Geometry check sheet. Reference: the model listing, model coordinates, mm. Face numbers are marked on the shaded views. A direction names the side the tool comes from. Round coordinates to 2 decimals unless told otherwise and drop trailing zeros. Order: outer loops, then holes, each group sorted by start corner. A loop starts at its lowest first (then second) coordinate and runs counter-clockwise, first axis right, second up. Notation, with made-up numbers: (20.5, -31.5) - (37.5, -31.5) arc R15 ccw to (37.5, -9.5) - close; hole circle Ø10 at (2.5, 82). An arc over 180 degrees is marked (long way). Use a Markdown table: item, result. Add a question column.
(1) Section check A-A on x = 28.25. Record the boundary of the cut face in (y, z) (3 decimals), then the cut area to 3 significant figures.
(2) Section check C-C on z = 13. Record the boundary of the cut face in (x, y), then the cut area to 3 significant figures.
(3) Section check D-D on z = 2.5. Record the boundary of the cut face in (x, y).
(4) Gauge pin test, flat ends, axial feed: P1, Ø3.5, axis at y = 15.5, z = -2, coming from the -X side; P2, Ø10.5, axis at y = -5.5, z = 20, coming from the -X side; P3, Ø6, axis at y = -18, z = 2, coming from the +X side; P4, Ø3, axis at x = 0, y = 0, coming from the -Z side. Record the tip position at first contact, or that the pin passes through.
(5) Access from +Z, -Z, +X, -X, +Y, -Y to the whole of each face (thin tool, end or side, straight path). Record for the marked faces 1, 2, 3 and 4.
(6) Thickness scan on line 1 along Y through (x, z) = (0, -1.3) (3 decimals); line 2 along Z through (x, y) = (-16.5, -10); line 3 along X through (y, z) = (-1, 4). Record the ranges inside material, lowest first. Write a range as [from, to].
```python
from build123d import *

# Parameters (mm, degrees)
F0_R     = 1
F0_R_2   = 1.25
F0_R_3   = 4.2
F0_R_4   = 1.275
F0_W     = 11.2
F0_H     = 6.2
F1_DEPTH = 3
F4_W     = 10.83598
F4_H     = 10.83598
F5_DEPTH = 40


with BuildPart() as f1:
    # F0 (on Top) → F1 (new body)
    with BuildSketch(Plane.XY):
        with BuildLine():
            ThreePointArc((26.336773, -20), (31.34153, -10.551499), (33.070011, 0))
            ThreePointArc((33.070011, 0), (14.700772, 29.622845), (-20, 26.336773))
            Line((-20, 26.336773), (-20, -20))
            Line((-20, -20), (26.336773, -20))
        make_face()
        with Locations((-15, 3e-06)):
            Circle(F0_R, mode=Mode.SUBTRACT)
        Circle(F0_R_2, mode=Mode.SUBTRACT)
        with Locations((0, 19)):
            Circle(F0_R_3, mode=Mode.SUBTRACT)
        with Locations((0, 28.25)):
            Circle(F0_R_4, mode=Mode.SUBTRACT)
        with Locations((11.580758, 16.082448)):
            Rectangle(F0_W, F0_H, mode=Mode.SUBTRACT)
        with Locations((28.25, 0)):
            Circle(F0_R_4, mode=Mode.SUBTRACT)
        with BuildLine():
            Line((-20, -20), (-20, 26.336773))
            ThreePointArc((-20, 26.336773), (-23.384029, -23.384029), (26.336773, -20))
            Line((26.336773, -20), (-20, -20))
        make_face()
        with Locations((-28.25, 0)):
            Circle(F0_R_4, mode=Mode.SUBTRACT)
    extrude(amount=-F1_DEPTH)

    # F2 (on Right) → F3 (revolve)
    with BuildSketch(Plane.YZ):
        Polygon((10, 0), (0, 37), (0, 0), align=None)
    revolve(axis=Axis((0, 0, 18.5), (0, 0, -1)))

    # F4 (on Top) → F5 (cut)
    with BuildSketch(Plane.XY):
        with Locations((-5.91799, 5.91799)):
            Rectangle(F4_W, F4_H)
        with Locations((5.91799, 5.91799)):
            Rectangle(F4_W, F4_H)
        with Locations((5.91799, -5.91799)):
            Rectangle(F4_W, F4_H)
        with Locations((-5.91799, -5.91799)):
            Rectangle(F4_W, F4_H)
    extrude(amount=F5_DEPTH, mode=Mode.SUBTRACT)


solid = f1.part
```
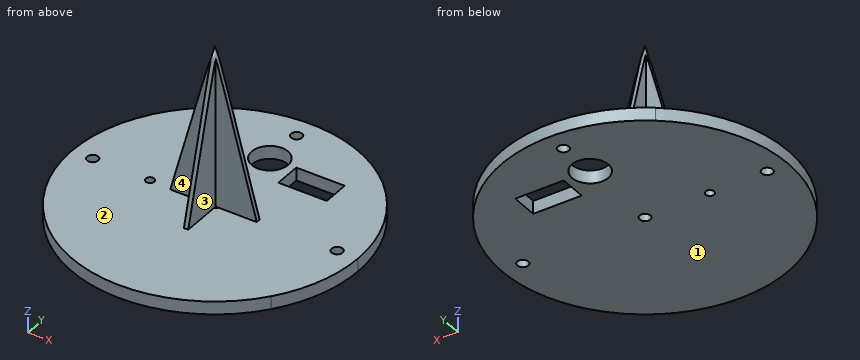
Check sheet entries:
| question | item | result |
|---|---|---|
| 1 | outline | (-17.192, -3) - (-1.275, -3) - (-1.275, 0) - (-17.192, 0) - close; (1.275, -3) - (17.192, -3) - (17.192, 0) - (1.275, 0) - close |
| 1 | area | 95.5 mm2 |
| 2 | outline | (-6.47, -0.5) - (-0.5, -0.5) - (-0.5, -6.47) arc R6.49 ccw to (0.5, -6.47) - (0.5, -0.5) - (6.47, -0.5) arc R6.49 ccw to (6.47, 0.5) - (0.5, 0.5) - (0.5, 6.47) arc R6.49 ccw to (-0.5, 6.47) - (-0.5, 0.5) - (-6.47, 0.5) arc R6.49 ccw to start |
| 2 | area | 24.9 mm2 |
| 3 | outline | (-9.31, -0.5) - (-0.5, -0.5) - (-0.5, -9.31) arc R9.32 ccw to (0.5, -9.31) - (0.5, -0.5) - (9.31, -0.5) arc R9.32 ccw to (9.31, 0.5) - (0.5, 0.5) - (0.5, 9.31) arc R9.32 ccw to (-0.5, 9.31) - (-0.5, 0.5) - (-9.31, 0.5) arc R9.32 ccw to start |
| 4 | P1 | stops at x = -30.08 |
| 4 | P2 | stops at x = -5 |
| 4 | P3 | stops at x = 29.07 |
| 4 | P4 | stops at z = -3 |
| 5 | face 1 | -Z, +X, -X, +Y, -Y |
| 5 | face 2 | +Z |
| 5 | face 3 | +Z, +X, -Y |
| 5 | face 4 | +Z, -X, -Y |
| 6 | line 1 | y = [-33.07, -1.25], [1.25, 14.8], [23.2, 26.975], [29.525, 33.07] |
| 6 | line 2 | z = [-3, 0] |
| 6 | line 3 | x = [-0.5, 0.5] |
